Design review of the part built by this model. Coordinates are the model's own, in mm. A direction names the side the tool comes from. Coordinates: 2 decimals unless noted, no trailing zeros. Loops run counter-clockwise (first coordinate to the right, second up) from the corner with the lowest first, then second, coordinate; pieces in that order, holes last. Notation, with made-up numbers: M 79,71.25 L 93,71.25 A25 ccw 93,99.25 Z; hole C 72.5,-35 d3. An arc over 180 degrees is marked long. Write item = value, one per line. Start each with the question number.
from build123d import *

# Parameters (mm, degrees)
F1_DEPTH = 70
F3_D     = 5
F3_DEPTH = 20
F3_TIP   = 1.5021515476
F5_D     = 5
F5_DEPTH = 15
F5_TIP   = 1.5021515476
F8_D     = 7
F8_DEPTH = 20
F8_TIP   = 2.1030121666


with BuildPart() as f1:
    # F0 (on Front) → F1 (new body, symmetric)
    with BuildSketch(Plane.XZ):
        Polygon((0, -20), (0, 10), (-27.5, 10), (-27.5, 0), (-17.5, 0), (-17.5, -20), align=None)
    extrude(amount=F1_DEPTH, both=True)

    # F3
    with Locations(Plane.XZ.offset(70)):
        with Locations((-10.5, 3), (-10.5, -13)):
            Hole(F3_D / 2, depth=F3_DEPTH)
            with Locations((0, 0, -(F3_DEPTH + F3_TIP / 2))):  # 118° drill point
                Cone(0, F3_D / 2, F3_TIP, mode=Mode.SUBTRACT)

    # F5
    with Locations(Plane(origin=(0, 0, -20), x_dir=(1, 0, 0), z_dir=(0, 0, -1))):
        with Locations((-12.5, 45), (-12.5, 0), (-12.5, -45)):
            Hole(F5_D / 2, depth=F5_DEPTH)
            with Locations((0, 0, -(F5_DEPTH + F5_TIP / 2))):  # 118° drill point
                Cone(0, F5_D / 2, F5_TIP, mode=Mode.SUBTRACT)

    # F6: F1 across plane


with BuildPart() as f1_1:
    add(f1.part)
    add(f1.part.mirror(Plane.YZ))

    # F8
    with Locations(Plane(origin=(0, 70, 0), x_dir=(-1, 0, 0), z_dir=(0, 1, 0))):
        with Locations((-10.5, 3), (10.5, 3), (0, -12)):
            Hole(F8_D / 2, depth=F8_DEPTH)
            with Locations((0, 0, -(F8_DEPTH + F8_TIP / 2))):  # 118° drill point
                Cone(0, F8_D / 2, F8_TIP, mode=Mode.SUBTRACT)


solid = f1_1.part
Q1. To check wall thickness, follow line 1 (X direction, y = 45, z = -14); line 2 (X direction, y = -62.25, z = -13); line 3 (Z direction, x = -10.5, y = 60.25). State the ranges of each line that lie inside material, in increasing order. Write a range as from..to.
Q2. Mouldability with a two-part tool opening along X and no side actions: class faces 4 (the face through (9.94, 48.26, 2.77)), 5 (the face through (-17.5, -1, -10)), 6 (the face through (-23, -1, 0)), 7 (the face through (-0.759, 59.86, -15.417)) as released by +X, released by -X, zero draft, split by the parting line, or undercut.
Q3. Add section C-C on x = 21. State the section outline as (y, z) points, plus the area to 3 significant figures.
Q4. Clearance check with flat-ended pins moving along their axes: P1, Ø12, axis at y = 37, z = -8.5, coming from the -X side; P2, Ø6, axis at y = 3, z = -10, coming from the +X side; P3, Ø6, axis at x = 21.5, z = -4, coming from the -Y side; P4, Ø11, axis at x = 0, z = -12, coming from the +Y side. State where each tip first meets the part, or that it passes through.
Q5. For faces 1 (the face through (-10.845, -48.759, -13.264)), 2 (the face through (11.96, 47.44, -12.4)), 3 (the face through (17.5, -1, -10)), list the 3-axis set-ups (+Z, -Z, +X, -X, +Y, -Y) from which the entire face can be reached by the end or side of a thin tool; tool diameter is ignored.
Q6. Add section B-B on y = -29. State the section outline as (x, z) points.
Q7. Add section A-A on z = -18. State the section outline as (x, y) points, plus the area to 3 significant figures.
Values follow:
q1.line_1 = -17.5..-15, -10..10, 15..17.5
q1.line_2 = -17.5..-13, -8..8, 13..17.5
q1.line_3 = -20..-0.5, 6.5..10
q2.face_4 = undercut
q2.face_5 = released by -X
q2.face_6 = zero draft
q2.face_7 = undercut
q3.outline = M -70,0 L 70,0 L 70,10 L -70,10 Z
q3.area = 1,400 mm2
q4.P1 = -17.5
q4.P2 = 17.5
q4.P3 = through
q4.P4 = 70
q5.face_1 = -Y
q5.face_2 = -Z
q5.face_3 = -Z, +X, +Y, -Y
q6.outline = M -27.5,0 L -17.5,0 L -17.5,-20 L 17.5,-20 L 17.5,0 L 27.5,0 L 27.5,10 L -27.5,10 Z
q7.outline = M -17.5,-70 L 17.5,-70 L 17.5,70 L -17.5,70 Z; hole C -12.5,-45 d5; hole C -12.5,0 d5; hole C -12.5,45 d5; hole C 12.5,-45 d5; hole C 12.5,0 d5; hole C 12.5,45 d5
q7.area = 4,780 mm2
